Solid Edge part; units mm, degrees
sketch "Sketch1" plane through (0, 0, 0) normal (0, 0, 1) x (1, 0, 0)
  circle A0 centre (29.3738, 16.8927) radius 15
extrude "Protrusion1" add sketch "Sketch1" along normal blind 140
sketch "Sketch2" plane through (29.3738, 16.8927, 140) normal (0, 0, 1) x (1, 0, 0)
  circle A0 centre (0, 0) radius 15
  circle A1 centre (0, 0) radius 12.5
extrude "ExtrudedCutout_1" cut sketch "Sketch2" against normal blind 32
sketch "Sketch3" plane through (29.3738, 16.8927, 140) normal (0, 0, 1) x (1, 0, 0)
  circle A0 centre (0, 0) radius 12.5
  circle A1 centre (0, 0) radius 10
extrude "ExtrudedCutout_2" cut sketch "Sketch3" against normal blind 20
sketch "Sketch4" plane through (29.3738, 16.8927, 0) normal (0, 0, -1) x (1, 0, 0)
  circle A0 centre (0, 0) radius 15
  circle A1 centre (0, 0) radius 12.5
extrude "Cutout1" cut sketch "Sketch4" against normal blind 58
sketch "Sketch5" plane through (29.3738, 16.8927, 0) normal (0, 0, -1) x (1, 0, 0)
  circle A0 centre (0, 0) radius 12.5
  circle A1 centre (0, 0) radius 10
extrude "ExtrudedCutout_4" cut sketch "Sketch5" against normal blind 46
sketch "Sketch6" plane through (29.3738, 16.8927, 0) normal (0, 0, -1) x (1, 0, 0)
  circle A0 centre (0, 0) radius 10
  circle A1 centre (0, 0) radius 7.5
extrude "ExtrudedCutout_5" cut sketch "Sketch6" against normal blind 16
sketch "Sketch7" plane through (29.3738, 16.8927, 140) normal (0, 0, 1) x (0, 1, 0)
  circle A0 centre (0, 0) radius 10
  circle A1 centre (0, 0) radius 5
extrude "ExtrudedCutout_6" cut sketch "Sketch7" against normal blind 20
sketch "Sketch8" plane through (29.3738, 16.8927, 120) normal (0, 0, 1) x (1, 0, 0)
  circle A0 centre (0, 0) radius 12.5
  circle A1 centre (0, 0) radius 7.5
extrude "Cutout2" cut sketch "Sketch8" against normal up to vertex (12 mm away)
sketch "Sketch9" plane through (29.3738, 16.8927, 0) normal (0, 0, -1) x (0, -1, 0)
  circle A0 centre (0, 0) radius 7.5
  circle A1 centre (0, 0) radius 5
extrude "Cutout3" cut sketch "Sketch9" against normal up to vertex (16 mm away)
sketch "Sketch10" plane through (29.3738, 16.8927, 16) normal (0, 0, -1) x (0, -1, 0)
  circle A0 centre (0, 0) radius 10
  circle A1 centre (0, 0) radius 7.5
extrude "ExtrudedCutout_12" cut sketch "Sketch10" against normal blind 30
sketch "Sketch11" plane through (29.3738, 16.8927, 46) normal (0, 0, -1) x (0, 1, 0)
  circle A0 centre (0, 0) radius 12.5
  circle A1 centre (0, 0) radius 10
extrude "Cutout4" cut sketch "Sketch11" against normal up to vertex (12 mm away)
Can you work these out from the model? Positions are in its coordinate system, mm. A direction names the side the tool comes from. Give positions to 0.01 mm unless a question says otherwise; leave off trailing zeros. Loops run counter-clockwise (first coordinate to the right, second up) from the corner with the lowest first, then second, coordinate; pieces in that order, holes last. Notation, with made-up numbers: M 35,-38.5 L 89,-38.5 A27 cw 89,-0.5 Z; hole C 10.5,39.25 d5. An arc over 180 degrees is marked long. One line per item, written item: value.
1) Please list where these lines run through material, in increasing order: line 1 (Z direction, x = 25, y = 20.5); line 2 (Z direction, x = 38, y = 13.25); line 3 (Y direction, x = 30.5, z = 107).
Geometry check:
line 1: z = 16 to 120
line 2: z = 46 to 108
line 3: y = 1.94 to 31.85
2) Imagine slicing it at D-D on x = 17. Write out the boundary of the cut face in (y, z).
Geometry check:
outline: M 8.41,58 L 25.37,58 L 25.37,108 L 8.41,108 Z
3) I'm going to push flat-ended pins straight in: pin 1 (6 mm diameter, centred on y = 28, z = 85, fed in from +X); pin 2 (1 mm diameter, centred on x = 27, y = 6, fed in from +Z); pin 3 (9 mm diameter, centred on x = 25.5, y = 9.5, fed in from +Z); pin 4 (5 mm diameter, centred on x = 33, z = 23, fed in from -Y). Where does each tip first touch, or does it pass through?
Geometry check:
pin 1: stops at x = 41.99
pin 2: stops at z = 108
pin 3: stops at z = 140
pin 4: stops at y = 9.48
4) Imagine slicing it at C-C on z = 49. Write out the boundary of the cut face in (x, y), and give its area (3 significant figures).
Geometry check:
outline: C 29.37,16.89 d20
area: 314 mm²
5) Imagine slicing it at B-B on y = 5.5. Write out the boundary of the cut face in (x, z), and give its area (3 significant figures).
Geometry check:
outline: M 19.62,58 L 39.13,58 L 39.13,108 L 19.62,108 Z
area: 976 mm²
6) On a 3-axis mill with a long thin cutter (end or side, diameter ignored), from which of +Z, -Z, +X, -X, +Y, -Y can I reach the whole of each face in a straight line? I mean faces 1 (the face through (22, 14, 108)), 2 (the face through (29, 17, 140)), 3 (the face through (32.246, 9.965, 30.79)). Say none if no direction works.
Geometry check:
face 1: +Z
face 2: +Z, +X, -X, +Y, -Y
face 3: -Z
7) Imagine slicing it at A-A on x = 31. Write out the boundary of the cut face in (y, z), and give its area (3 significant figures).
Geometry check:
outline: M 1.98,58 L 7.03,58 L 7.03,46 L 9.57,46 L 9.57,16 L 12.16,16 L 12.16,0 L 21.62,0 L 21.62,16 L 24.21,16 L 24.21,46 L 26.76,46 L 26.76,58 L 31.8,58 L 31.8,108 L 24.21,108 L 24.21,120 L 21.62,120 L 21.62,140 L 12.16,140 L 12.16,120 L 9.57,120 L 9.57,108 L 1.98,108 Z
area: 2,680 mm²
